from build123d import *

# Parameters (mm, degrees)
SKETCH_1_R          = 27
SKETCH_1_R_2        = 25.25
EXTRUDE_1_DEPTH     = 27
SKETCH_3_R          = 27
SKETCH_3_R_2        = 2.4
EXTRUDE_2_DEPTH     = 3
SKETCH_7_W          = 4
SKETCH_7_H          = 4
EXTRUDE_3_DEPTH     = 14
SKETCH_8_R          = 1.25
CUT_EXTRUDE_1_DEPTH = 14
SKETCH_10_W         = 4
SKETCH_10_H         = 10
EXTRUDE_4_DEPTH     = 14
SKETCH_11_R         = 2.5
CUT_EXTRUDE_3_DEPTH = 14
SKETCH_12_R         = 5
CUT_EXTRUDE_4_DEPTH = 14
SKETCH_13_R         = 2.4
CUT_EXTRUDE_5_DEPTH = 2
SKETCH_14_R         = 2.4
CUT_EXTRUDE_6_DEPTH = 91


with BuildPart() as part:
    # 草图1 → 凸台-拉伸1 (new body)
    with BuildSketch(Plane(origin=(0, 0, 0), x_dir=(1, 0, 0), z_dir=(0, 1, 0))):
        Circle(SKETCH_1_R)
        Circle(SKETCH_1_R_2, mode=Mode.SUBTRACT)
    extrude(amount=EXTRUDE_1_DEPTH)

    # 草图3 → 凸台-拉伸2 (add)
    with BuildSketch(Plane(origin=(0, 27, 0), x_dir=(1, 0, 0), z_dir=(0, 1, 0))):
        Circle(SKETCH_3_R)
        Circle(SKETCH_3_R_2, mode=Mode.SUBTRACT)
    extrude(amount=EXTRUDE_2_DEPTH)

    # 草图5 → 旋转2 (revolve)
    with BuildSketch(Plane.XY):
        Polygon((27, 30), (31.564027788, 0), (27, 0), align=None)
    revolve(axis=Axis((0, 0, 0), (0, 1, 0)))

    # 草图7 → 凸台-拉伸3 (add)
    with BuildSketch(Plane(origin=(0, 30, 0), x_dir=(1, 0, 0), z_dir=(0, 1, 0))):
        with Locations((-9, 19)):
            Rectangle(SKETCH_7_W, SKETCH_7_H)
        with Locations((-9, -8)):
            Rectangle(SKETCH_7_W, SKETCH_7_H)
    extrude(amount=EXTRUDE_3_DEPTH)

    # 草图8 → 切除-拉伸1 (cut)
    with BuildSketch(Plane(origin=(-7, 0, 0), x_dir=(0, 0, -1), z_dir=(1, 0, 0))):
        with Locations((-8, 40)):
            Circle(SKETCH_8_R)
        with Locations((19, 40)):
            Circle(SKETCH_8_R)
    extrude(amount=-CUT_EXTRUDE_1_DEPTH, mode=Mode.SUBTRACT)

    # 草图10 → 凸台-拉伸4 (add)
    with BuildSketch(Plane(origin=(0, 30, 0), x_dir=(1, 0, 0), z_dir=(0, 1, 0))):
        with Locations((16, 0)):
            Rectangle(SKETCH_10_W, SKETCH_10_H)
    extrude(amount=EXTRUDE_4_DEPTH)

    # 草图11 → 切除-拉伸3 (cut)
    with BuildSketch(Plane(origin=(18, 0, 0), x_dir=(0, 0, -1), z_dir=(1, 0, 0))):
        with Locations((0, 40)):
            Circle(SKETCH_11_R)
    extrude(amount=-CUT_EXTRUDE_3_DEPTH, mode=Mode.SUBTRACT)

    # 草图12 → 切除-拉伸4 (cut)
    with BuildSketch(Plane(origin=(0, 30, 0), x_dir=(1, 0, 0), z_dir=(0, 1, 0))):
        with Locations((0, -15.04505665)):
            Circle(SKETCH_12_R)
    extrude(amount=-CUT_EXTRUDE_4_DEPTH, mode=Mode.SUBTRACT)

    # 草图13 → 切除-拉伸5 (cut)
    with BuildSketch(Plane(origin=(0, 30, 0), x_dir=(1, 0, 0), z_dir=(0, 1, 0))):
        with BuildLine():
            Line((-2.610752853, 2.331087631), (-15, 2))
            ThreePointArc((-15, 2), (-16.999822183, 0.026669038), (-15.053333333, -1.999288762))
            Line((-15.053333333, -1.999288762), (-2.610641885, -2.331211906))
            ThreePointArc((-2.610641885, -2.331211906), (3.499999999, 8.3304e-05), (-2.610752853, 2.331087631))
        make_face()
        Circle(SKETCH_13_R, mode=Mode.SUBTRACT)
    extrude(amount=-CUT_EXTRUDE_5_DEPTH, mode=Mode.SUBTRACT)

    # 草图14 → 切除-拉伸6 (cut)
    with BuildSketch(Plane(origin=(0, 28, 0), x_dir=(1, 0, 0), z_dir=(0, 1, 0))):
        with BuildLine():
            ThreePointArc((-2.610752853, 2.331087631), (-3.499999999, -8.3304e-05), (-2.610641885, -2.331211906))
            ThreePointArc((-2.610641885, -2.331211906), (1.247548276, -3.270110594), (3.5, 0))
            ThreePointArc((3.5, 0), (1.247470444, 3.270140286), (-2.610752853, 2.331087631))
        make_face()
        Circle(SKETCH_14_R, mode=Mode.SUBTRACT)
    extrude(amount=-CUT_EXTRUDE_6_DEPTH, mode=Mode.SUBTRACT)


solid = part.part
Geometry check sheet. Reference: the model listing, model coordinates, mm. A direction names the side the tool comes from. Give positions to 0.01 mm unless a question says otherwise; leave off trailing zeros. Write each loop counter-clockwise with the first axis right and the second up, starting at its lowest first coordinate (ties: lowest second). Pieces come first, ordered by that corner, then holes. Notation, with made-up numbers: (37.5, -17.5) - (77.5, -17.5) arc R31 ccw to (77.5, 10.5) - close; hole circle Ø9 at (38.5, 67.5). An arc over 180 degrees is marked (long way). Put each result on its own line as item: value.
1. Sectioned sample at B-B, the plane x = 0. Enter the section's corners in (y, z), plus the area to 3 significant figures.
Ans:
outline: (0, -31.56) - (30, -27) - (30, -3.5) - (27, -3.5) - (27, -25.25) - (0, -25.25) - close; (0, 25.25) - (27, 25.25) - (27, 20.05) - (30, 20.05) - (30, 27) - (0, 31.56) - close; (27, 3.5) - (30, 3.5) - (30, 10.05) - (27, 10.05) - close
area: 342 mm²
2. Draft check along X on faces 5 (the cylindrical face through (-5.47, 13.31, 24.65)), 6 (the flat face through (-24, 0, 9)), 7 (the flat face through (-7, 37, -19)). Enter one of: +X half, -X half, draft (parallel to the pull), parting line (faces both ways), or undercut.
Ans:
face 5: undercut
face 6: draft
face 7: +X half
3. Sectioned sample at D-D, the plane y = 5.5. Enter the section's corners in (x, z), plus the area to 3 significant figures.
Ans:
outline: circle Ø61.45 at (0, 0); hole circle Ø50.5 at (0, 0)
area: 963 mm²
4. Thickness scan on line 1 (Y direction, x = -8, z = -19); line 2 (Y direction, x = -15.5, z = -22); line 3 (X direction, y = 19.5, z = 13). Record the ranges inside material, lowest first.
Ans:
line 1: y = 27 to 38.75, 41.25 to 44
line 2: y = 0 to 30
line 3: x = -25.47 to -21.65, 21.65 to 25.47
5. Go/stop test with flat-tipped pins: pin 1 (4 mm diameter, centred on y = 18.5, z = 5.5, fed in from -X); pin 2 (4 mm diameter, centred on x = -4, y = 8, fed in from +Z); pin 3 (1.5 mm diameter, centred on y = 40, z = 8, fed in from +X); pin 4 (3 mm diameter, centred on y = 40, z = -19, fed in from -X). Record where each tip stops, or that it passes through.
Ans:
pin 1: stops at x = -28.68
pin 2: stops at z = 30.46
pin 3: passes through
pin 4: stops at x = -11
6. Set-up check for faces 1 (the flat face through (-9, 37, -17)), 2 (the flat face through (16, 37, -5)), 3 (the flat face through (5, 27, 0)), 4 (the flat face through (-11, 37, 8)): record each of +Z, -Z, +X, -X, +Y, -Y from which the full face is reachable in a straight line by a thin tool's end or side.
Ans:
face 1: +X, -X, +Y
face 2: -Z, +X, -X, +Y
face 3: -Y
face 4: +Z, -Z, -X, +Y
7. Sectioned sample at C-C, the plane y = 32. Enter the section's corners in (x, z), plus the area to 3 significant figures.
Ans:
outline: (-11, -21) - (-7, -21) - (-7, -17) - (-11, -17) - close; (-11, 6) - (-7, 6) - (-7, 10) - (-11, 10) - close; (14, -5) - (18, -5) - (18, 5) - (14, 5) - close
area: 72.0 mm²
8. Sectioned sample at A-A, the plane y = 40. Enter the section's corners in (x, z).
Ans:
outline: (-11, -21) - (-7, -21) - (-7, -20.25) - (-11, -20.25) - close; (-11, -17.75) - (-7, -17.75) - (-7, -17) - (-11, -17) - close; (-11, 6) - (-7, 6) - (-7, 6.75) - (-11, 6.75) - close; (-11, 9.25) - (-7, 9.25) - (-7, 10) - (-11, 10) - close; (14, -5) - (18, -5) - (18, -2.5) - (14, -2.5) - close; (14, 2.5) - (18, 2.5) - (18, 5) - (14, 5) - close
